Could you check a few things on this model? Use its own coordinates, in mm. Give positions to 0.01 mm unless a question says otherwise; leave off trailing zeros. Order: outer loops, then holes, each group sorted by start corner. A loop starts at its lowest first (then second) coordinate and runs counter-clockwise, first axis right, second up. Notation, with made-up numbers: (-40, 82) - (-15, 82) arc R17 ccw to (-15, 89) - close; hole circle Ø10 at (27, -12). An arc over 180 degrees is marked (long way). One line per question, with ' | ' between items. Start each with the question number.
1. I need wall thicknesses on probe 1 along X at (y, z) = (2.5, 0); probe 2 along X at (y, z) = (7, 0); probe 3 along X at (y, z) = (1, 1.5). Which ranges of each line are inside material? Lowest first, please. Write a range as from..to.
2. If we mould it in two halves opening along Z, with no side actions, what happens to faces 1 (the flat face through (0, 0, 0)), 2 (the cylindrical face through (13.715, 5.07, 4.699)), 3 (the cylindrical face through (12, 5, 0))? For each: released by +Z, released by -Z, zero draft, split by the parting line, or undercut.
3. Imagine slicing it at C-C (z = -0.5). Please give me the cut outline in (x, y), and give its area (3 significant figures).
4. For P1, Ø5, axis at x = -0.5, z = -3.5, coming from the +Y side; P2, Ø4, axis at x = -6, z = 2, coming from the -Y side, each with a flat end and sliding along its axis, tell me the tip position at first contact or that it passes through.
5. Imagine slicing it at B-B (y = 8.75). Please give me the cut outline in (x, z), and give its area (3 significant figures).
6. Imagine slicing it at D-D (y = 5.75). Please give me the cut outline in (x, z), and give its area (3 significant figures).
7. Imagine slicing it at A-A (x = -10). Please give me the cut outline in (y, z).
```python
from build123d import *

# Parameters (mm, degrees)
BOSS_EXTRUDE1_DEPTH = 5
CUT_EXTRUDE1_REACH  = 19.916
SKETCH4_R           = 2
FILLET1_R           = 1


with BuildPart() as part:
    # Sketch1 → Boss-Extrude1 (new, symmetric)
    with BuildSketch(Plane.XY):
        with BuildLine():
            Line((-14, 0), (14, 0))
            Line((14, 0), (14, 10))
            Line((14, 10), (6.5, 10))
            ThreePointArc((6.5, 10), (0, 3.5), (-6.5, 10))
            Line((-6.5, 10), (-14, 10))
            Line((-14, 10), (-14, 0))
        make_face()
    extrude(amount=BOSS_EXTRUDE1_DEPTH, both=True)

    # Sketch2 → Cut-Revolve2 (revolve, cut)
    with BuildSketch(Plane.XY):
        Polygon((-2.748441557, 5.239559582), (-7.60591541, -3.173831928), (-8.688447164, -2.548831928), (-3.830973311, 5.864559582), align=None)
    revolve(axis=Axis((-2.748441557, 5.239559582, 0), (-0.4999999999999947, -0.8660254037844417, 0)), mode=Mode.SUBTRACT)

    # Sketch4 → Cut-Extrude1 (cut, up to next)
    with BuildSketch(Plane(origin=(0, 10, 0), x_dir=(1, 0, 0), z_dir=(0, 1, 0)), mode=Mode.PRIVATE) as cut_extrude1_sk1:
        with Locations(Location((-10, 0, 0), (0, 0, 270))):
            Circle(SKETCH4_R)
    cut_extrude1_tool1 = extrude(cut_extrude1_sk1.sketch, amount=-CUT_EXTRUDE1_REACH, mode=Mode.PRIVATE) & part.part
    # Sketch4 → Cut-Extrude1 (cut, up to next)
    with BuildSketch(Plane(origin=(0, 10, 0), x_dir=(1, 0, 0), z_dir=(0, 1, 0)), mode=Mode.PRIVATE) as cut_extrude1_sk2:
        with Locations(Location((10, 0, 0), (0, 0, 270))):
            Circle(SKETCH4_R)
    cut_extrude1_tool2 = extrude(cut_extrude1_sk2.sketch, amount=-CUT_EXTRUDE1_REACH, mode=Mode.PRIVATE) & part.part
    add(cut_extrude1_tool1.solids().sort_by_distance((-10, 10, 0))[0], mode=Mode.SUBTRACT)
    add(cut_extrude1_tool2.solids().sort_by_distance((10, 10, 0))[0], mode=Mode.SUBTRACT)

    # Fillet1
    fillet1_edges = [part.edges().sort_by_distance(p)[0] for p in [
        (14, 5, 5),
        (-14, 5, 5),
        (14, 5, -5),
        (-14, 5, -5),
    ]]
    fillet(fillet1_edges, radius=FILLET1_R)


solid = part.part
```
Results found:
1) probe 1: x = -14..-12, -8..-5.77, -2.89..8, 12..14 | probe 2: x = -14..-12, -8..-5.77, 5.77..8, 12..14 | probe 3: x = -14..-11.32, -8.68..8.68, 11.32..14
2) face 1: zero draft | face 2: released by +Z | face 3: undercut
3) outline: (-14, 0) - (-11.94, 0) - (-11.94, 10) - (-14, 10) - close; (-8.06, 0) - (-7.1, 0) - (-4.19, 5.03) arc R6.5 cw to (-6.5, 10) - (-8.06, 10) - close; (-4.45, 0) - (8.06, 0) - (8.06, 10) - (6.5, 10) arc R6.5 cw to (-2.21, 3.89) - close; (11.94, 0) - (14, 0) - (14, 10) - (11.94, 10) - close | area: 125 mm2
4) P1: stops at y = 4.23 | P2: stops at y = 0
5) outline: (-14, -4) arc R1 ccw to (-13, -5) - (-6.38, -5) - (-6.38, 5) - (-13, 5) arc R1 ccw to (-14, 4) - close; (6.38, -5) - (13, -5) arc R1 ccw to (14, -4) - (14, 4) arc R1 ccw to (13, 5) - (6.38, 5) - close; hole circle Ø4 at (-10, 0); hole circle Ø4 at (10, 0) | area: 126 mm2
6) outline: (-14, -4) arc R1 ccw to (-13, -5) - (-4.92, -5) - (-4.92, 5) - (-13, 5) arc R1 ccw to (-14, 4) - close; (4.92, -5) - (13, -5) arc R1 ccw to (14, -4) - (14, 4) arc R1 ccw to (13, 5) - (4.92, 5) - close; hole circle Ø4 at (-10, 0); hole circle Ø4 at (10, 0) | area: 156 mm2
7) outline: (0, -5) - (10, -5) - (10, -2) - (0, -2) - close; (0, 2) - (10, 2) - (10, 5) - (0, 5) - close
